The figure shows three views and two pictorial views of one solid part (mm, origin at its lowest corner). Answer the questions. A direction names the side the tool comes from. Coordinates: 2 decimals unless noted, no trailing zeros. Loops run counter-clockwise (first coordinate to the right, second up) from the corner with the lowest first, then second, coordinate; pieces in that order, holes last. Notation, with made-up numbers: (-17.75, 44.25) -> (39.25, 44.25) arc R18 ccw to (39.25, 48.25) -> close; hole circle Ø10 at (-25, 89.25). An arc over 180 degrees is marked (long way). Use a Markdown table: item, result. Add a question column.
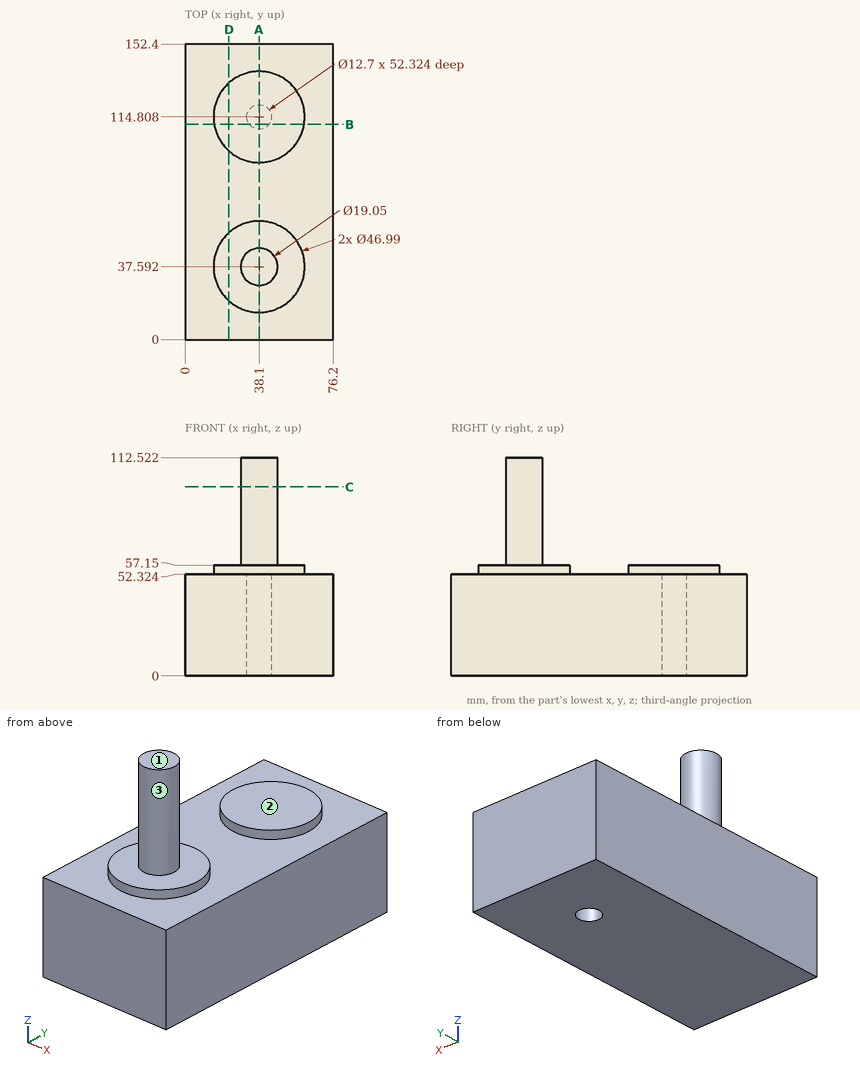
Item 1: Section D-D (x = 22.5) is taken. Determine the outline of the cut face in (y, z), then the cut area to 3 significant figures.
Item 2: Find the intervals of material crossed by probe 1 along Y at (x, z) = (38.1, 40); probe 2 along Z at (x, y) = (49.5, 51.5); probe 3 along Z at (x, y) = (38, 75), in increasing order.
Item 3: Section B-B (y = 111) is taken. Determine the outline of the cut face in (x, z), then the cut area to 3 significant figures.
Item 4: Section A-A (x = 38.1) is taken. Determine the outline of the cut face in (y, z).
Item 5: For the marked faces 1, 2 and 3, determine the directions among +Z, -Z, +X, -X, +Y, -Y from which every point of the face is accessible in a straight line to the end or side of a thin tool.
Item 6: Given pin 1 (23 mm diameter, centred on x = 42.5, y = 101, fed in from +Z); pin 2 (8 mm diameter, centred on y = 52.5, z = 101, fed in from +X); pin 3 (6.5 mm diameter, centred on x = 36.5, y = 114, fed in from -Z); pin 4 (5 mm diameter, centred on x = 38.5, z = 84, fed in from -Y), each flat-ended and moving along its own axis, determine where each tip first touches the part or whether it passes through.
Item 7: Section C-C (z = 97.5) is taken. Determine the outline of the cut face in (x, y) (3 decimals).
Output:
| question | item | result |
|---|---|---|
| 1 | outline | (0, 0) -> (152.4, 0) -> (152.4, 52.32) -> (132.38, 52.32) -> (132.38, 57.15) -> (97.24, 57.15) -> (97.24, 52.32) -> (55.16, 52.32) -> (55.16, 57.15) -> (20.02, 57.15) -> (20.02, 52.32) -> (0, 52.32) -> close |
| 1 | area | 8,310 mm2 |
| 2 | probe 1 | y = 0 to 108.46, 121.16 to 152.4 |
| 2 | probe 2 | z = 0 to 57.15 |
| 2 | probe 3 | z = 0 to 52.32 |
| 3 | outline | (0, 0) -> (33.02, 0) -> (33.02, 52.32) -> (43.18, 52.32) -> (43.18, 0) -> (76.2, 0) -> (76.2, 52.32) -> (61.28, 52.32) -> (61.28, 57.15) -> (14.92, 57.15) -> (14.92, 52.32) -> (0, 52.32) -> close |
| 3 | area | 3,680 mm2 |
| 4 | outline | (0, 0) -> (108.46, 0) -> (108.46, 52.32) -> (121.16, 52.32) -> (121.16, 0) -> (152.4, 0) -> (152.4, 52.32) -> (138.3, 52.32) -> (138.3, 57.15) -> (91.31, 57.15) -> (91.31, 52.32) -> (61.09, 52.32) -> (61.09, 57.15) -> (47.12, 57.15) -> (47.12, 112.52) -> (28.07, 112.52) -> (28.07, 57.15) -> (14.1, 57.15) -> (14.1, 52.32) -> (0, 52.32) -> close |
| 5 | face 1 | +Z, +X, -X, +Y, -Y |
| 5 | face 2 | +Z, +X, -X, +Y |
| 5 | face 3 | +Z |
| 6 | pin 1 | stops at z = 57.15 |
| 6 | pin 2 | passes through |
| 6 | pin 3 | stops at z = 52.32 |
| 6 | pin 4 | stops at y = 28.07 |
| 7 | outline | circle Ø19.05 at (38.1, 37.592) |
